from build123d import *

# Parameters (mm, degrees)
F0_R     = 10.0040416518
F1_DEPTH = 7.04


with BuildPart() as f1:
    # F0 (on Top) → F1 (new body)
    with BuildSketch(Plane.XY):
        with BuildLine():
            ThreePointArc((8.0596013479, 39.4250795937), (18.9862113581, 26.931715548), (9.3900539463, 13.3896066124))
            ThreePointArc((9.3900539463, 13.3896066124), (12.8029919773, 10.175366076), (15.1637771231, 6.1249115676))
            Line((15.1637771231, 6.1249115676), (15.937639911, 6.1249115676))
            Line((15.937639911, 6.1249115676), (28.0554961826, 6.1249115676))
            ThreePointArc((28.0554961826, 6.1249115676), (33.4743323204, 8.3717454292), (38.2599624573, 4.9791370399))
            ThreePointArc((38.2599624573, 4.9791370399), (35.9003199694, 33.3723310432), (8.0596013479, 39.4250795937))
        make_face()
        with BuildLine():
            ThreePointArc((35.4391843293, 16.2098441298), (29.4013015143, 15.8466192988), (24.3793946911, 12.4749115676))
            Line((24.3793946911, 12.4749115676), (19.7612497114, 12.4749115676))
            ThreePointArc((19.7612497114, 12.4749115676), (25.0400123396, 22.7411647393), (23.6803165677, 34.204694583))
            ThreePointArc((23.6803165677, 34.204694583), (32.6253176497, 27.2104868561), (35.4391843293, 16.2098441298))
        make_face(mode=Mode.SUBTRACT)
        with BuildLine():
            ThreePointArc((15.1637771231, 6.1249115676), (12.8029919773, 10.175366076), (9.3900539463, 13.3896066124))
            ThreePointArc((9.3900539463, 13.3896066124), (-2.1364828918, 16.2138866162), (-12.5379799884, 10.5001779109))
            ThreePointArc((-12.5379799884, 10.5001779109), (-14.9968569617, 6.5229563558), (-16.2297438327, 2.0124844036))
            ThreePointArc((-16.2297438327, 2.0124844036), (-13.0647635418, -9.8370031995), (-2.5516255591, -16.1537576234))
            ThreePointArc((-2.5516255591, -16.1537576234), (-2.5484818112, -16.154253892), (-2.5453379668, -16.1547495488))
            ThreePointArc((-2.5453379668, -16.1547495488), (-2.5451208542, -16.1547837555), (-2.5449037412, -16.1548179593))
            ThreePointArc((-2.5449037412, -16.1548179593), (2.1768059123, -16.2085222759), (6.717037457, -14.9109384732))
            ThreePointArc((6.717037457, -14.9109384732), (13.7350898923, -8.877048158), (16.3540416518, 0))
            ThreePointArc((16.3540416518, 0), (16.0537179653, 3.1197464384), (15.1637771231, 6.1249115676))
        make_face()
        Circle(F0_R, mode=Mode.SUBTRACT)
        with BuildLine():
            ThreePointArc((-16.2297438327, 2.0124844036), (-14.9968569617, 6.5229563558), (-12.5379799884, 10.5001779109))
            Line((-12.5379799884, 10.5001779109), (-13.1381993498, 11.348302759))
            Line((-13.1381993498, 11.348302759), (-18.6180223097, 19.38283416))
            ThreePointArc((-18.6180223097, 19.38283416), (-22.886896, 22.8371620642), (-22.2051291736, 28.2860938723))
            ThreePointArc((-22.2051291736, 28.2860938723), (-44.431743107, 11.8873369712), (-36.4311702867, -14.5499932531))
            ThreePointArc((-36.4311702867, -14.5499932531), (-32.9169731903, 1.7648878816), (-16.2297438327, 2.0124844036))
        make_face()
        with BuildLine():
            ThreePointArc((-27.8425738277, 20.8345445104), (-26.5172228087, 18.8430269716), (-24.8001450054, 17.1773915828))
            Line((-24.8001450054, 17.1773915828), (-20.4118380564, 10.7432439401))
            ThreePointArc((-20.4118380564, 10.7432439401), (-30.7174803102, 10.1222622456), (-39.3025332707, 4.3873911753))
            ThreePointArc((-39.3025332707, 4.3873911753), (-36.142247382, 14.4014653535), (-27.8425738277, 20.8345445104))
        make_face(mode=Mode.SUBTRACT)
        with BuildLine():
            ThreePointArc((28.3540401584, -27.7120920045), (13.0814706801, -28.8399527249), (6.717037457, -14.9109384732))
            ThreePointArc((6.717037457, -14.9109384732), (2.1768059123, -16.2085222759), (-2.5449037412, -16.1548179593))
            ThreePointArc((-2.5449037412, -16.1548179593), (-2.5451208542, -16.1547837555), (-2.5453379668, -16.1547495488))
            ThreePointArc((-2.5453379668, -16.1547495488), (-2.5484818112, -16.154253892), (-2.5516255591, -16.1537576234))
            Line((-2.5516255591, -16.1537576234), (-3.4641944059, -17.2808545138))
            Line((-3.4641944059, -17.2808545138), (-9.8543521959, -27.576888898))
            ThreePointArc((-9.8543521959, -27.576888898), (-11.0679351896, -32.9167573694), (-16.4773315191, -33.7684676051))
            ThreePointArc((-16.4773315191, -33.7684676051), (8.0897637018, -46.6657507467), (28.3540401584, -27.7120920045))
        make_face()
        with BuildLine():
            ThreePointArc((-5.9789437938, -36.7808810105), (-3.8125370617, -33.0947145568), (-3.1808303734, -28.8659927744))
            Line((-3.1808303734, -28.8659927744), (0.8243466838, -22.4127185282))
            ThreePointArc((0.8243466838, -22.4127185282), (6.3485406517, -31.6703504661), (15.9104272307, -36.6493858287))
            ThreePointArc((15.9104272307, -36.6493858287), (4.9886650126, -40.5310640467), (-5.9789437938, -36.7808810105))
        make_face(mode=Mode.SUBTRACT)
    extrude(amount=F1_DEPTH)


solid = f1.part
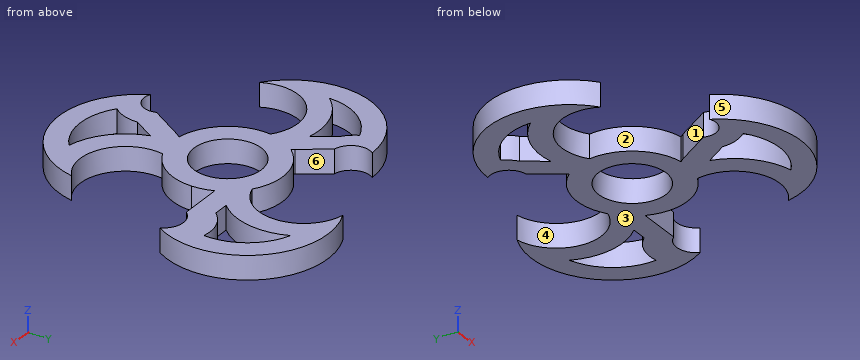
CAD build for the part. Positions are in the model's coordinates, mm. Face numbers are marked on the shaded views. A direction names the side the tool comes from. Give positions to 0.01 mm unless a question says otherwise; leave off trailing zeros. Loops run counter-clockwise (first coordinate to the right, second up) from the corner with the lowest first, then second, coordinate; pieces in that order, holes last. Notation, with made-up numbers: M 74.25,-16.5 L 101.25,-16.5 A30 ccw 101.25,12.5 Z; hole C 42,72 d5. An arc over 180 degrees is marked long. Answer in a Markdown table with one row per item. Add a question column.
Item 1: Probe probe 1 along Y at (x, z) = (0, 4); probe 2 along Y at (x, z) = (2, 0.75); probe 3 along X at (y, z) = (6.5, 6.25). List the from-to ranges inside material, lowest first.
Item 2: Band-saw the part on A-A on x = -33. Give the cut face in (y, z), then the cut area to 3 significant figures.
Item 3: Band-saw the part on D-D on x = 30. Give the cut face in (y, z), then the cut area to 3 significant figures.
Item 4: Band-saw the part on C-C on z = 3. Give the number of separate pieces and of enclosed holes in the cut face, then the cut area to 3 significant figures.
Item 5: Tool access for the marked faces 4, 5 and 6: list every direction of +Z, -Z, +X, -X, +Y, -Y with a clear straight run to the whole face (end or side of a thin tool).
Item 6: Band-saw the part on B-B on y = 25. Give the cut face in (x, z), then the cut area to 3 significant figures.
Item 7: Mould opens along X. For the marked faces 1, 2 and 3 say: +X half, -X half, draft (parallel to the pull), parting line (faces both ways), or undercut.
Item 8: Drop flat-ended pins along their axis: P1, Ø3.5, axis at x = 21.5, z = 2.5, coming from the +Y side; P2, Ø1, axis at y = 5.5, z = 1.5, coming from the +X side; P3, Ø2, axis at x = 32.5, z = 2.5, coming from the +Y side. Give the stop position or say it passes through.
Reply:
| question | item | result |
|---|---|---|
| 1 | probe 1 | y = -46.38 to -39.84, -23.74 to -10, 10 to 16.35 |
| 1 | probe 2 | y = -46.71 to -40.29, -25.65 to -9.8, 9.8 to 16.23 |
| 1 | probe 3 | x = -45.55 to -39.17, -37.15 to -7.6, 7.6 to 28.38, 37.22 to 39.13 |
| 2 | outline | M 1.7,0 L 9.19,0 L 9.19,7.04 L 1.7,7.04 Z; M 17.83,0 L 25.46,0 L 25.46,7.04 L 17.83,7.04 Z |
| 2 | area | 106 mm^2 |
| 3 | outline | M 7.73,0 L 16.03,0 L 16.03,7.04 L 7.73,7.04 Z; M 30.36,0 L 38.25,0 L 38.25,7.04 L 30.36,7.04 Z |
| 3 | area | 114 mm^2 |
| 4 | separate pieces | 1 |
| 4 | enclosed holes | 4 |
| 4 | area | 2,290 mm^2 |
| 5 | face 4 | +Z, -Z |
| 5 | face 5 | +Z, -Z, -Y |
| 5 | face 6 | +Z, -Z, +Y |
| 6 | outline | M -33.82,0 L -23.3,0 L -23.3,7.04 L -33.82,7.04 Z; M 18.95,0 L 25.31,0 L 25.31,7.04 L 18.95,7.04 Z; M 33.85,0 L 40.66,0 L 40.66,7.04 L 33.85,7.04 Z |
| 6 | area | 167 mm^2 |
| 7 | face 1 | -X half |
| 7 | face 2 | undercut |
| 7 | face 3 | draft |
| 8 | P1 | stops at y = 41.46 |
| 8 | P2 | stops at x = 38.86 |
| 8 | P3 | stops at y = 37.29 |
